from build123d import *

# Parameters (mm, degrees)
BOSS_EXTRU_1_DEPTH = 500
BOSS_EXTRU_3_DEPTH = 600


with BuildPart() as part:
    # Esquisse1 → Boss.-Extru.1 (new body)
    with BuildSketch(Plane.XY):
        Polygon((0, 0), (500, 0), (500, 100), (300, 100), (300, 1000), (200, 1000), (200, 100), (0, 100), align=None)
    extrude(amount=BOSS_EXTRU_1_DEPTH)

    # Esquisse4 → Boss.-Extru.3 (add)
    with BuildSketch(Plane(origin=(0, 100, 0), x_dir=(1, 0, 0), z_dir=(0, 1, 0))):
        Polygon((200, -80), (200, -130), (190, -130), (190, -100), (185, -100), (185, -130), (175, -130), (175, -80), align=None)
        Polygon((175, -370), (175, -420), (200, -420), (200, -370), (190, -370), (190, -400), (185, -400), (185, -370), align=None)
    extrude(amount=BOSS_EXTRU_3_DEPTH)


solid = part.part
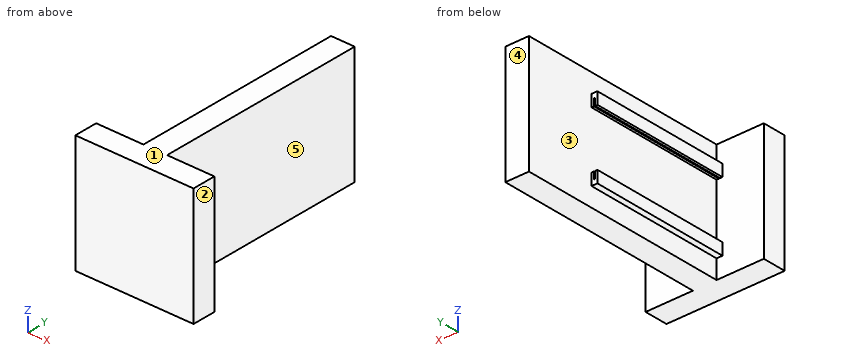
Design review of the part built by this model. Coordinates are the model's own, in mm. Face numbers are marked on the shaded views. A direction names the side the tool comes from. Coordinates: 2 decimals unless noted, no trailing zeros. Loops run counter-clockwise (first coordinate to the right, second up) from the corner with the lowest first, then second, coordinate; pieces in that order, holes last. Notation, with made-up numbers: (-11.75, 50) -> (41.25, 50) arc R22 ccw to (41.25, 87) -> close; hole circle Ø11 at (54.5, 31.25). An arc over 180 degrees is marked (long way). Use a Markdown table: item, result. Add a question column.
Item 1: Wall thickness on L1, parallel to X at y = 112, z = 102.5; L2, parallel to Y at x = 450.5, z = 232; L3, parallel to X at y = 157.5, z = 341.5: over which ranges is each line inside the solid? List them lowest first. Write a range as from..to.
Item 2: Clearance check with flat-ended pins moving along their axes: P1, Ø9, axis at y = 310, z = 121, coming from the +X side; P2, Ø3, axis at y = 646.5, z = 146, coming from the -X side; P3, Ø24, axis at y = 426.5, z = 384, coming from the -X side. State where each tip first meets the part, or that it passes through.
Item 3: We need section A-A, the plane z = 201.5. Write out the cut boundary in (x, y).
Item 4: We need section D-D, the plane y = 864.5. Write out the cut boundary in (x, z).
Item 5: The part is to be moulded in two halves that separate along Z. For the marked faces 1, 2 and 3, say which applies: +Z half, -Z half, draft (parallel to the pull), parting line (faces both ways), or undercut.
Item 6: Machinability: for the marked faces 4 and 5, which of the approach directions +Z, -Z, +X, -X, +Y, -Y give a long, thin tool a straight path to every point of the face, cutting with its end or side? Answer none if there is none.
Item 7: We need section B-B, the plane y = 527. Write out the cut boundary in (x, z), and give its area (3 significant figures).
Item 8: We need section C-C, the plane x = 138. Write out the cut boundary in (y, z).
Numbers:
| question | item | result |
|---|---|---|
| 1 | L1 | x = 175..185, 190..300 |
| 1 | L2 | y = 0..100 |
| 1 | L3 | x = 200..300 |
| 2 | P1 | stops at x = 300 |
| 2 | P2 | stops at x = 200 |
| 2 | P3 | stops at x = 175 |
| 3 | outline | (0, 0) -> (500, 0) -> (500, 100) -> (300, 100) -> (300, 1000) -> (200, 1000) -> (200, 100) -> (0, 100) -> close |
| 4 | outline | (200, 0) -> (300, 0) -> (300, 500) -> (200, 500) -> close |
| 5 | face 1 | +Z half |
| 5 | face 2 | draft |
| 5 | face 3 | undercut |
| 6 | face 4 | +Z, -Z, +X, -X, +Y |
| 6 | face 5 | +Z, -Z, +X, +Y |
| 7 | outline | (175, 80) -> (200, 80) -> (200, 0) -> (300, 0) -> (300, 500) -> (200, 500) -> (200, 420) -> (175, 420) -> (175, 370) -> (185, 370) -> (185, 400) -> (190, 400) -> (190, 370) -> (200, 370) -> (200, 130) -> (190, 130) -> (190, 100) -> (185, 100) -> (185, 130) -> (175, 130) -> close |
| 7 | area | 52,200 mm^2 |
| 8 | outline | (0, 0) -> (100, 0) -> (100, 500) -> (0, 500) -> close |
